Study the drawing (mm; zero at the part's minimum x, y, z) and answer. Coordinates: 2 decimals unless noted, no trailing zeros. Write each loop counter-clockwise with the first axis right and the second up, starting at its lowest first coordinate (ties: lowest second). Pieces come first, ordered by that corner, then holes. Notation, with made-up numbers: (41.25, 25.5) -> (60.25, 25.5) arc R18 ccw to (60.25, 51.5) -> close; hole circle Ø10 at (34, 58.25). An arc over 180 degrees is marked (long way). Answer in a Markdown table with one row per item. Add a question column.
Item 1: Section B-B on y = 121 is taken. Write down the section's boundary in (x, z), then the cut area to 3 significant figures.
Item 2: Section C-C on x = 45 is taken. Write down the section's boundary in (y, z).
Item 3: Straight lines are drawn through the part: line 1 (Y direction, x = 47, z = 1.75); line 2 (X direction, y = 143.5, z = 1.95). For each, find the intervals that lie inside material, in ascending order. Write a range as from..to.
Item 4: Given pin 1 Ø1 at (y, z) = (48, 1.5) entering from +X; pin 2 Ø0.6 at (x, z) = (52.5, 1) entering from +Y; pin 3 Ø1 at (y, z) = (127.5, 1) entering from -X, each flat-ended and moving along its own axis, determine where each tip first touches the part or whether it passes through.
Item 5: Section A-A on z = 1.2 is taken. Write down the section's boundary in (x, y), then the cut area to 3 significant figures.
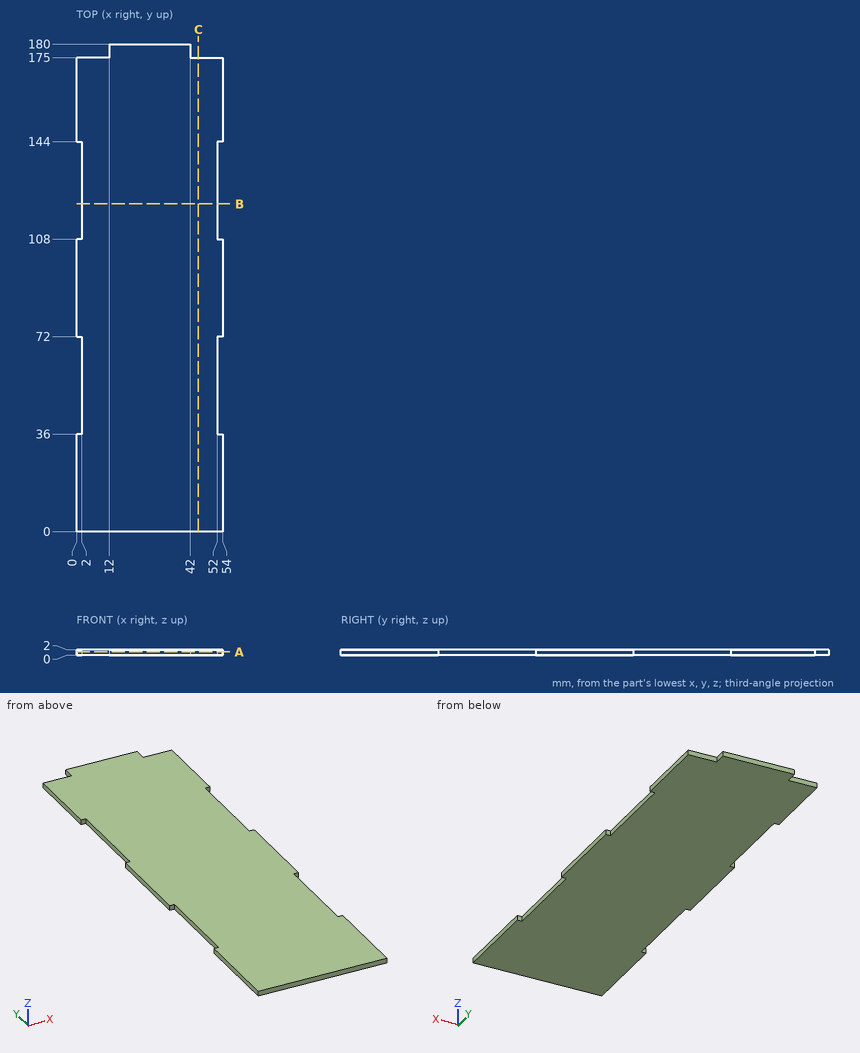
Results below:
| question | item | result |
|---|---|---|
| 1 | outline | (2, 0) -> (52, 0) -> (52, 2) -> (2, 2) -> close |
| 1 | area | 100 mm2 |
| 2 | outline | (0, 0) -> (175, 0) -> (175, 2) -> (0, 2) -> close |
| 3 | line 1 | y = 0..175 |
| 3 | line 2 | x = 2..52 |
| 4 | pin 1 | stops at x = 52 |
| 4 | pin 2 | stops at y = 175 |
| 4 | pin 3 | stops at x = 2 |
| 5 | outline | (0, 0) -> (54, 0) -> (54, 36) -> (52, 36) -> (52, 72) -> (54, 72) -> (54, 108) -> (52, 108) -> (52, 144) -> (54, 144) -> (54, 175) -> (42, 175) -> (42, 180) -> (12, 180) -> (12, 175) -> (0, 175) -> (0, 144) -> (2, 144) -> (2, 108) -> (0, 108) -> (0, 72) -> (2, 72) -> (2, 36) -> (0, 36) -> close |
| 5 | area | 9,310 mm2 |
